Source: three-view drawing plus pictorial views. Frame: mm from the lowest corner of the part. Give positions to 0.01 mm unless a question says otherwise; leave off trailing zeros. Order: outer loops, then holes, each group sorted by start corner. A loop starts at its lowest first (then second) coordinate and runs counter-clockwise, first axis right, second up. Notation, with made-up numbers: (-12.5, -25.5) -> (41.5, -25.5) arc R6 cw to (41.5, -18.5) -> close; hole circle Ø3 at (4.5, 41.25). An arc over 180 degrees is marked (long way). Answer in a Markdown table with one row per item. Add a question column.
Q1. Contact query for flat-ended pins moving along their axis: P1, Ø1.5, axis at x = 89, y = 33.5, coming from the -Z side; P2, Ø3, axis at x = 48.5, y = 34.5, coming from the +Z side. Output: stop coordinate, or through.
Q2. Cut plane B-B on y = 35. Return the cut outline in (x, z).
Q3. Line query: line 1 along Y through (x, z) = (50, 15); line 2 along Y through (x, z) = (50, 32.3); line 3 along Z through (x, y) = (53, 33.5). Output: solid intervals per line, ascending. Write a range as from..to.
Q4. Pull-direction query (X, two-part tool) for the marked faces 1, 2 and 3; classes: +X half, -X half, draft (parallel to the pull), parting line (faces both ways), or undercut.
Q5. Cut plane A-A on x = 50. Return the cut outline in (y, z).
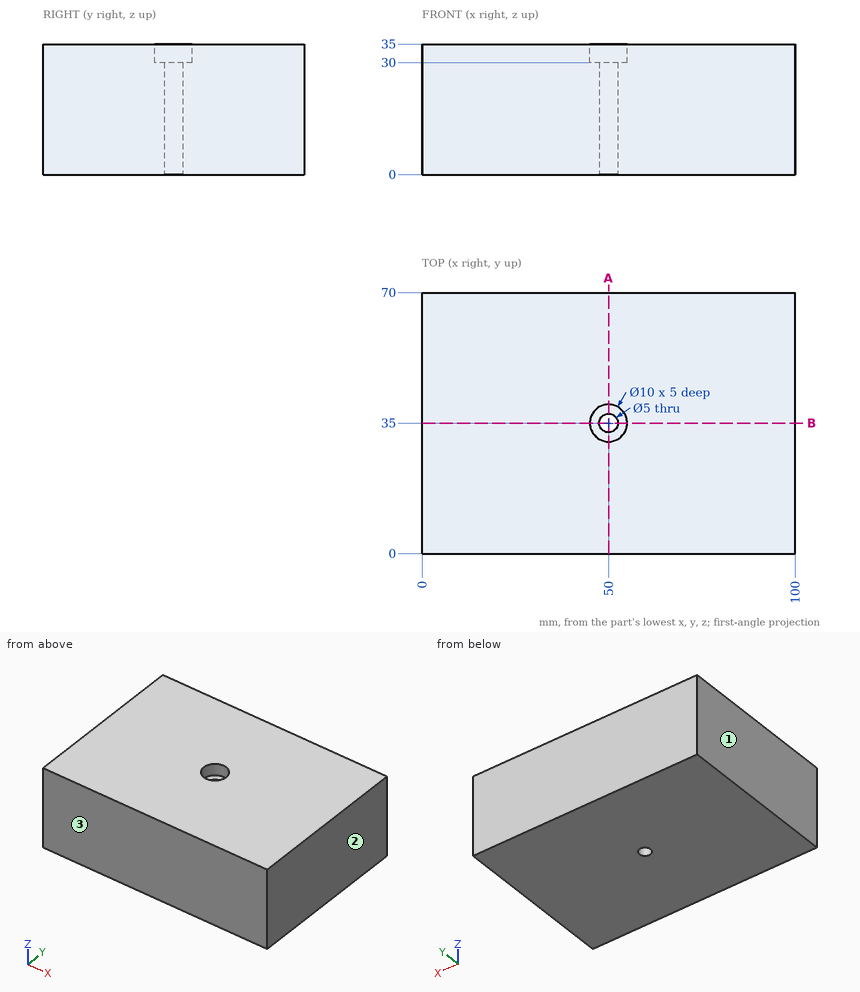
Completed:
| question | item | result |
|---|---|---|
| 1 | P1 | stops at z = 0 |
| 1 | P2 | stops at z = 30 |
| 2 | outline | (0, 0) -> (47.5, 0) -> (47.5, 30) -> (45, 30) -> (45, 35) -> (0, 35) -> close; (52.5, 0) -> (100, 0) -> (100, 35) -> (55, 35) -> (55, 30) -> (52.5, 30) -> close |
| 3 | line 1 | y = 0..32.5, 37.5..70 |
| 3 | line 2 | y = 0..30, 40..70 |
| 3 | line 3 | z = 0..30 |
| 4 | face 1 | -X half |
| 4 | face 2 | +X half |
| 4 | face 3 | draft |
| 5 | outline | (0, 0) -> (32.5, 0) -> (32.5, 30) -> (30, 30) -> (30, 35) -> (0, 35) -> close; (37.5, 0) -> (70, 0) -> (70, 35) -> (40, 35) -> (40, 30) -> (37.5, 30) -> close |
